Work out the finished part from the listing and answer in its coordinate system (mm). A direction names the side the tool comes from. Give positions to 0.01 mm unless a question says otherwise; leave off trailing zeros. Order: outer loops, then holes, each group sorted by start corner. A loop starts at its lowest first (then second) coordinate and runs counter-clockwise, first axis right, second up. Notation, with made-up numbers: M -35,-22 L -17,-22 A30 ccw -17,5 Z; hole C -21.75,49 d6. An arc over 180 degrees is marked long. One line per item, written item: value.
from build123d import *

# Parameters (mm, degrees)
F0_W           = 10
F0_H           = 10
F1_DEPTH       = 32
F2_R           = 3
F3_DEPTH       = 52
F4_R           = 2.5
F5_DEPTH       = 12.5
F6_SIZE        = 1
F7_R           = 0.5
F8_R           = 0.75
F9_R           = 9
F10_DEPTH      = 25
F10_TAPER      = -10
F10_DEPTH_BACK = 25
F10_TAPER_BACK = 10


with BuildPart() as f1:
    # F0 (on Right) → F1 (new body, symmetric)
    with BuildSketch(Plane.YZ):
        Rectangle(F0_W, F0_H)
    extrude(amount=F1_DEPTH, both=True)

    # F2 (on Right) → F3 (join, symmetric)
    with BuildSketch(Plane.YZ):
        Circle(F2_R)
    extrude(amount=F3_DEPTH, both=True)

    # F4 (on Top) → F5 (cut, symmetric)
    with BuildSketch(Plane.XY):
        Circle(F4_R)
    extrude(amount=F5_DEPTH, both=True, mode=Mode.SUBTRACT)

    # F6
    f6_edges = [f1.edges().sort_by_distance(p)[0] for p in [
        (52, -3, 0),
        (-52, -3, 0),
    ]]
    chamfer(f6_edges, length=F6_SIZE)

    # F7
    f7_edges = [f1.edges().sort_by_distance(p)[0] for p in [
        (0, -5, 5),
        (0, 5, 5),
        (0, -5, -5),
        (0, 5, -5),
        (-32, 5, 0),
        (-32, 0, -5),
        (32, 0, -5),
        (-2.5, 0, -5),
        (-32, -5, 0),
        (-32, 0, 5),
        (32, 0, 5),
        (32, -5, 0),
        (32, 5, 0),
    ]]
    fillet(f7_edges, radius=F7_R)

    # F8
    f8_edges = [f1.edges().sort_by_distance(p)[0] for p in [
        (32, -3, 0),
        (-32, -3, 0),
    ]]
    fillet(f8_edges, radius=F8_R)

    # F9 (on Front) → F10 (cut, two sides)
    with BuildSketch(Plane.XZ) as f10_sk:
        with Locations((0, 12)):
            Circle(F9_R)
    extrude(amount=F10_DEPTH, taper=F10_TAPER, mode=Mode.SUBTRACT)
    extrude(f10_sk.sketch, amount=-F10_DEPTH_BACK, taper=F10_TAPER_BACK, mode=Mode.SUBTRACT)


solid = f1.part
(1) Given P1, Ø2.5, axis at y = -1, z = -2, coming from the +X side; P2, Ø2, axis at y = -2.5, z = -2.5, coming from the +X side, each flat-ended and moving along its own axis, determine where each tip first touches the part or whether it passes through.
Findings:
P1: stops at x = 52
P2: stops at x = 51.46
(2) Section D-D, the plane x = 36 is taken. Give the vertices of the cut face in (y, z).
Findings:
outline: C 0,0 d6
(3) Section B-B, the plane x = 0 is taken. Give the vertices of the cut face in (y, z), then the cut area to 3 significant figures.
Findings:
outline: M -5,-4.5 A0.5 ccw -4.5,-5 L -3,-5 A0.5 ccw -2.5,-4.5 L -2.5,2.56 L -5,2.12 Z; M 2.5,-4.5 A0.5 ccw 3,-5 L 4.5,-5 A0.5 ccw 5,-4.5 L 5,3.88 L 2.5,3.44 Z
area: 39.8 mm^2
(4) Determine the mould class of faces 1 (the conical face through (-1.71, -2.15, 2.78)), 2 (the cylindrical face through (42, -3, 0)), 3 (the cylindrical face through (1.34, 2.11, -0.45)), 4 (the flat face through (-32, -4, 0)) for opening direction Y: pulls with the +Y half, pulls with the -Y half, needs draft (parallel to the pull), parting line crosses it, or undercut.
Findings:
face 1: pulls with the -Y half
face 2: parting line crosses it
face 3: undercut
face 4: needs draft
(5) Section A-A, the plane z = 0 is taken. Give the vertices of the cut face in (x, y).
Findings:
outline: M -52,-2 L -51,-3 L -32.75,-3 A0.75 cw -32,-3.75 L -32,-4.5 A0.5 ccw -31.5,-5 L 31.5,-5 A0.5 ccw 32,-4.5 L 32,-3.75 A0.75 cw 32.75,-3 L 51,-3 L 52,-2 L 52,2 L 51,3 L 32.75,3 A0.75 cw 32,3.75 L 32,4.5 A0.5 ccw 31.5,5 L -31.5,5 A0.5 ccw -32,4.5 L -32,3.75 A0.75 cw -32.75,3 L -51,3 L -52,2 Z; hole C 0,0 d5
(6) Which of the six approach directions +Z, -Z, +X, -X, +Y, -Y give full straight-line access (tool end or side, diameter ignored) to faces 5 (the flat face through (52, 0, 0)), 6 (the cylindrical face through (-42, -3, 0)), 7 (the flat face through (32, -4, 0))?
Findings:
face 5: +Z, -Z, +X, +Y, -Y
face 6: -X
face 7: +X
(7) Find the intervals of material crossed by probe 1 along X at (y, z) = (0, 1.25); probe 2 along Y at (x, z) = (1.5, -2); probe 3 along Y at (x, z) = (0, -1.5), in increasing order. Write a range as from..to.
Findings:
probe 1: x = -52..-2.5, 2.5..52
probe 2: y = -5..-2, 2..5
probe 3: y = -5..-2.5, 2.5..5
